Verification items for the finished model (mm, model axes). A direction names the side the tool comes from. Give positions to 0.01 mm unless a question says otherwise; leave off trailing zeros. Loops run counter-clockwise (first coordinate to the right, second up) from the corner with the lowest first, then second, coordinate; pieces in that order, holes last. Notation, with made-up numbers: (83, 42) -> (98, 42) arc R27 ccw to (98, 58) -> close; hole circle Ø7 at (52, 24). An arc over 180 degrees is marked (long way). Use one line per item in the form item = value. Start each with the question number.
from build123d import *

# Parameters (mm, degrees)
F3_DEPTH      = 3
F3_DEPTH_BACK = 3
F5_DEPTH      = 5
F5_DEPTH_BACK = 5
F6_SCALE      = 1.5


with BuildPart() as f2:
    # F0 (on Front) → F2 (revolve)
    with BuildSketch(Plane.XZ):
        with BuildLine():
            Line((-25, 5), (-15.0003286976, 5.0810792445))
            ThreePointArc((-15.0003286976, 5.0810792445), (-20.040703971, 10.0403752734), (-25, 5))
        make_face()
    revolve(axis=Axis((-20.0001643488, 0, 5.0405396222), (0.9999671302, 0, 0.0081079244)))

    # F0 (on Front) → F3 (join, two sides)
    with BuildSketch(Plane.XZ) as f3_sk:
        with BuildLine():
            ThreePointArc((-23.2302926299, -0.6269286958), (-22.8623688248, -0.1714255301), (-22.3024899558, 0))
            Line((-22.3024899558, 0), (0, 0))
            Line((0, 0), (0, 2))
            Line((0, 2), (-24.5, 2))
            ThreePointArc((-24.5, 2), (-24.8535533906, 1.8535533906), (-25, 1.5))
            Line((-25, 1.5), (-25, 0.0967607601))
            ThreePointArc((-25, 0.0967607601), (-25.0091076144, 0.0017625194), (-25.036098663, -0.089774892))
            Line((-25.036098663, -0.089774892), (-26.9623704714, -4.8802803922))
            ThreePointArc((-26.9623704714, -4.8802803922), (-26.9127563693, -5.3467554788), (-26.4984691344, -5.5668160443))
            Line((-26.4984691344, -5.5668160443), (-25.5544878752, -5.5668160443))
            ThreePointArc((-25.5544878752, -5.5668160443), (-25.2745484408, -5.4811032792), (-25.0905865382, -5.2533516964))
            Line((-25.0905865382, -5.2533516964), (-23.2302926299, -0.6269286958))
        make_face()
    extrude(amount=-F3_DEPTH)
    extrude(f3_sk.sketch, amount=F3_DEPTH_BACK)

    # F4: F2 across plane


with BuildPart() as f2_1:
    add(f2.part)
    add(f2.part.mirror(Plane.YZ))

    # F1 (on Right) → F5 (join, two sides)
    with BuildSketch(Plane.YZ) as f5_sk:
        with BuildLine():
            Line((-7.6333043873, 0), (0, 0))
            Line((0, 0), (0, 2))
            Line((0, 2), (-5.1333043873, 2))
            ThreePointArc((-5.1333043873, 2), (-5.8404111685, 2.2928932188), (-6.1333043873, 3))
            Line((-6.1333043873, 3), (-6.1333043873, 7))
            ThreePointArc((-6.1333043873, 7), (-5.8404111685, 7.7071067812), (-5.1333043873, 8))
            Line((-5.1333043873, 8), (-1.6333043873, 8))
            ThreePointArc((-1.6333043873, 8), (-0.9261976061, 8.2928932188), (-0.6333043873, 9))
            ThreePointArc((-0.6333043873, 9), (-0.9261976061, 9.7071067812), (-1.6333043873, 10))
            Line((-1.6333043873, 10), (-7.6333043873, 10))
            ThreePointArc((-7.6333043873, 10), (-8.3404111685, 9.7071067812), (-8.6333043873, 9))
            Line((-8.6333043873, 9), (-8.6333043873, 1))
            ThreePointArc((-8.6333043873, 1), (-8.3404111685, 0.2928932188), (-7.6333043873, 0))
        make_face()
    extrude(amount=F5_DEPTH)
    extrude(f5_sk.sketch, amount=-F5_DEPTH_BACK)


with BuildPart() as f2_2:
    # F6: moved
    add(f2_1.part.scale(F6_SCALE).moved(Location((-2.5, 0.8166521937, -5))))


solid = f2_2.part
Item 1: Sectioned sample at A-A, the plane x = -26. Enter the section's corners in (y, z), and give its area (3 significant figures).
Item 2: Gauge pin test, flat ends, axial feed: pin 1 Ø5 at (x, z) = (-11, 6.5) entering from +Y; pin 2 Ø10 at (y, z) = (-3, -2.5) entering from -X; pin 3 Ø1.5 at (x, y) = (-6, 1.5) entering from +Z. Record the tip position at first contact, or that the pin passes through.
Item 3: Sectioned sample at C-C, the plane x = -5.5. Enter the section's corners in (y, z).
Item 4: Sectioned sample at D-D, the plane y = -9.5. Enter the section's corners in (x, z).
Item 5: Tool access check on faces 4 (the flat face through (23, -3.683, -4)), 5 (the flat face through (-40, 1, -4)), 6 (the flat face through (35, 1, -4)). Record the directions out of +Z, -Z, +X, -X, +Y, -Y that give a thin tool (end or side, any length) a straight path to the whole face; none if there is none.
Item 6: Draft check along Z on faces 1 (the flat face through (-39, 1, -2)), 2 (the flat face through (-42, 1, -13.35)), 3 (the flat face through (-2, 5.317, -4)). Enter one of: +Z half, -Z half, draft (parallel to the pull), parting line (faces both ways), or undercut.
Item 7: Sectioned sample at B-B, the plane y = -5.5. Enter the section's corners in (x, z), and give its area (3 significant figures).
Item 8: Material ranges on line 1 (Z direction, x = 0.5, y = -3.5); line 2 (Z direction, x = 13.5, y = 3.5); line 3 (X direction, y = 2, z = 2), recorded low to high.
Outcome:
q1.outline = (-3.68, -5) -> (5.32, -5) -> (5.32, -2) -> (-3.68, -2) -> close; circle Ø7.48 at (0.82, 2.56)
q1.area = 71.0 mm^2
q2.pin_1 = -0.13
q2.pin_2 = -41.01
q2.pin_3 = -2
q3.outline = (-12.13, -3.5) arc R1.5 ccw to (-10.63, -5) -> (5.32, -5) -> (5.32, -2) -> (-6.88, -2) arc R1.5 cw to (-8.38, -0.5) -> (-8.38, 5.5) arc R1.5 cw to (-6.88, 7) -> (-1.63, 7) arc R1.5 ccw to (-1.63, 10) -> (-10.63, 10) arc R1.5 ccw to (-12.13, 8.5) -> close
q4.outline = (-10, -5) -> (5, -5) -> (5, 10) -> (-10, 10) -> close
q5.face_4 = -Z, -Y
q5.face_5 = +Z, -X, +Y, -Y
q5.face_6 = +Z, +X, +Y, -Y
q6.face_1 = undercut
q6.face_2 = -Z half
q6.face_3 = draft
q7.outline = circle Ø8.09 at (-32.5, 2.56); (-10, -5) -> (5, -5) -> (5, -2) -> (-10, -2) -> close; (-10, 7) -> (5, 7) -> (5, 10) -> (-10, 10) -> close; circle Ø8.09 at (27.5, 2.56)
q7.area = 193 mm^2
q8.line_1 = -5 to -2, 7 to 10
q8.line_2 = -5 to -2
q8.line_3 = -39.89 to -25.12, 20.12 to 34.89
